Could you check a few things on this drawing? It's one solid part, dimensions in mm from its lowest x, y, z. Round coordinates to 2 decimals unless told otherwise and drop trailing zeros. Write each loop counter-clockwise with the first axis right and the second up, starting at its lowest first coordinate (ties: lowest second). Pieces come first, ordered by that corner, then holes. Notation, with made-up numbers: M 25,83.25 L 74,83.25 A11 cw 74,98.25 Z; hole C -6,67 d10. An arc over 180 degrees is marked long. One line per item, written item: value. Start each with the question number.
(1) I want a section at A-A on x = 8.1. Please give me the cut outline in (y, z), and give its area (3 significant figures).
(2) If I drill on L1, parallel to Y at x = 8.1, z = 3.75; L2, parallel to Y at x = 4.75, z = 10 (1 decimal); L3, parallel to X at y = 8.5, z = 2.25, over which ranges is the centre line in solid material (lowest first)?
(3) I want a section at B-B on y = 8.1. Please give me the cut outline in (x, z), and give its area (3 significant figures).
(4) I'm going to push flat-ended pins straight in: pin 1 Ø2 at (y, z) = (4.5, 3.5) entering from -X; pin 2 Ø1 at (y, z) = (3.5, 8.5) entering from +X; pin 3 Ø1.5 at (x, z) = (6.5, 9) entering from -Y. Where does each tip first touch, or does it pass through?
(5) I want a section at C-C on x = 10. Please give me the cut outline in (y, z).
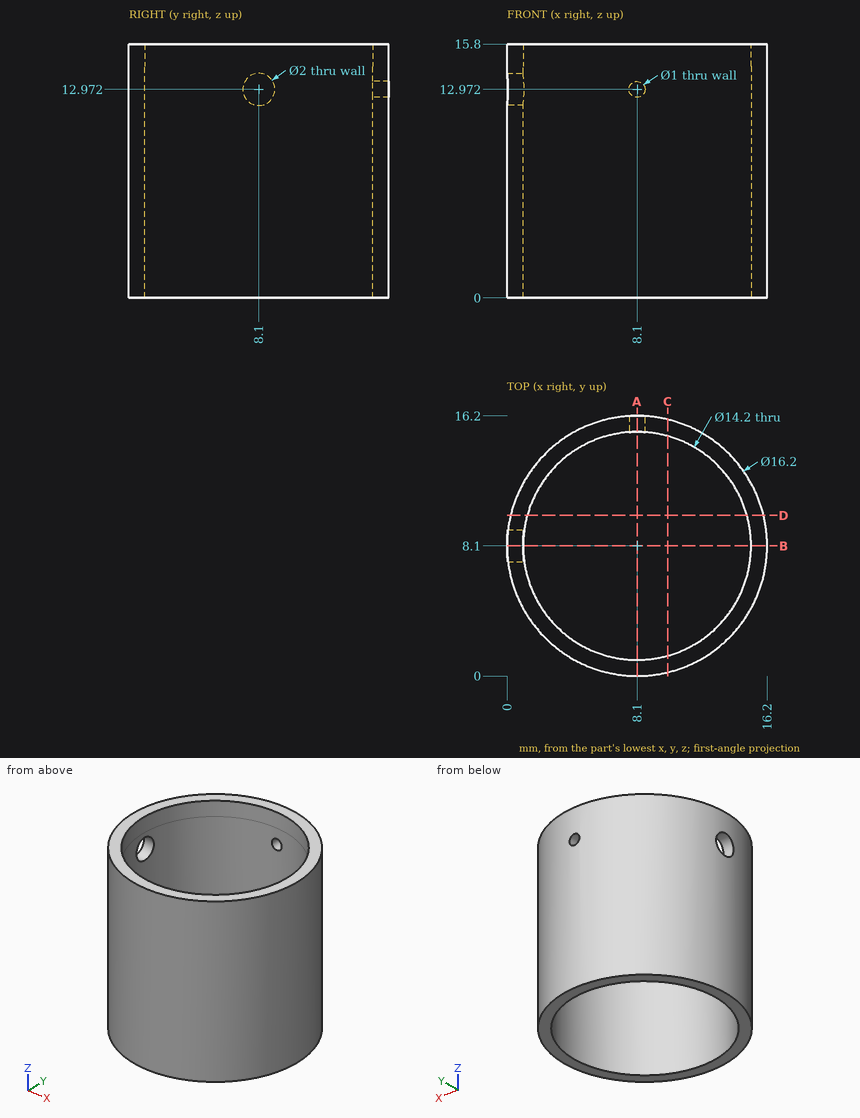
Found:
1. outline: M 0,0 L 1,0 L 1,15.8 L 0,15.8 Z; M 15.2,0 L 16.2,0 L 16.2,12.47 L 15.2,12.47 Z; M 15.2,13.47 L 16.2,13.47 L 16.2,15.8 L 15.2,15.8 Z
1. area: 30.6 mm²
2. L1: y = 0 to 1, 15.2 to 16.2
2. L2: y = 0.7 to 1.8, 14.4 to 15.5
2. L3: x = 0.01 to 1.01, 15.19 to 16.19
3. outline: M 0,0 L 1,0 L 1,11.97 L 0,11.97 Z; M 0,13.97 L 1,13.97 L 1,15.8 L 0,15.8 Z; M 15.2,0 L 16.2,0 L 16.2,15.8 L 15.2,15.8 Z
3. area: 29.6 mm²
4. pin 1: stops at x = 0.43
4. pin 2: stops at x = 15.09
4. pin 3: stops at y = 0.04
5. outline: M 0.23,0 L 1.26,0 L 1.26,15.8 L 0.23,15.8 Z; M 14.94,0 L 15.97,0 L 15.97,15.8 L 14.94,15.8 Z
